```python
from build123d import *

# Parameters (mm, degrees)
SKETCH1_R           = 41
SKETCH1_R_2         = 5
BOSS_EXTRUDE1_DEPTH = 3
SKETCH2_W           = 11
SKETCH2_H           = 12
BOSS_EXTRUDE2_DEPTH = 25
SKETCH3_W           = 7
SKETCH3_H           = 8
CUT_EXTRUDE1_DEPTH  = 65.389440128
SKETCH4_W           = 3
SKETCH4_H           = 3
CUT_EXTRUDE2_DEPTH  = 69.023892861
BOSS_EXTRUDE3_START = -7
BOSS_EXTRUDE3_DEPTH = 7
SKETCH6_R           = 10
SKETCH6_R_2         = 8
BOSS_EXTRUDE4_DEPTH = 5.5


with BuildPart() as part:
    # Sketch1 → Boss-Extrude1 (new body)
    with BuildSketch(Plane.XY):
        Circle(SKETCH1_R)
        Circle(SKETCH1_R_2, mode=Mode.SUBTRACT)
    extrude(amount=BOSS_EXTRUDE1_DEPTH)

    # Sketch2 → Boss-Extrude2 (add)
    with BuildSketch(Plane.XY.offset(3)):
        with Locations((0, 30)):
            Rectangle(SKETCH2_W, SKETCH2_H)
        with Locations((0, 15.301408404)):
            Rectangle(SKETCH2_W, SKETCH2_H)
    extrude(amount=BOSS_EXTRUDE2_DEPTH)

    # Sketch3 → Cut-Extrude1 (cut, through all)
    with BuildSketch(Plane.XY.offset(28)):
        with Locations((0, 30)):
            Rectangle(SKETCH3_W, SKETCH3_H)
        with Locations((0, 15.301408404)):
            Rectangle(SKETCH3_W, SKETCH3_H)
    extrude(amount=-CUT_EXTRUDE1_DEPTH, mode=Mode.SUBTRACT)

    # Sketch4 → Cut-Extrude2 (cut, through all)
    with BuildSketch(Plane(origin=(5.5, 0, 0), x_dir=(0, 0, -1), z_dir=(1, 0, 0))):
        with Locations((-22.5, 15.301408404)):
            Rectangle(SKETCH4_W, SKETCH4_H)
        with Locations((-22.5, 30)):
            Rectangle(SKETCH4_W, SKETCH4_H)
    extrude(amount=-CUT_EXTRUDE2_DEPTH, mode=Mode.SUBTRACT)

    # Sketch5 → Boss-Extrude3 (add)
    with BuildSketch(Plane.XY.offset(3).offset(BOSS_EXTRUDE3_START)):
        with BuildLine():
            Line((16.484910619, 42.944660385), (14.693085931, 38.276797486))
            ThreePointArc((14.693085931, 38.276797486), (20.5, 35.507041555), (25.802136033, 31.86298442))
            Line((25.802136033, 31.86298442), (28.948711541, 35.748681567))
            ThreePointArc((28.948711541, 35.748681567), (22.999978988, 39.837132179), (16.484910619, 42.944660385))
        make_face()
        with BuildLine():
            Line((45.43362216, 7.195978818), (40.495221964, 6.413813067))
            ThreePointArc((40.495221964, 6.413813067), (41, 0), (40.495221964, -6.413813067))
            Line((40.495221964, -6.413813067), (45.43362216, -7.195978818))
            ThreePointArc((45.43362216, -7.195978818), (45.999957975, 0), (45.43362216, 7.195978818))
        make_face()
        with BuildLine():
            Line((28.948711541, -35.748681567), (25.802136033, -31.86298442))
            ThreePointArc((25.802136033, -31.86298442), (20.5, -35.507041555), (14.693085931, -38.276797486))
            Line((14.693085931, -38.276797486), (16.484910619, -42.944660385))
            ThreePointArc((16.484910619, -42.944660385), (22.999978988, -39.837132179), (28.948711541, -35.748681567))
        make_face()
        with BuildLine():
            Line((-16.484910619, -42.944660385), (-14.693085931, -38.276797486))
            ThreePointArc((-14.693085931, -38.276797486), (-20.5, -35.507041555), (-25.802136033, -31.86298442))
            Line((-25.802136033, -31.86298442), (-28.948711541, -35.748681567))
            ThreePointArc((-28.948711541, -35.748681567), (-22.999978988, -39.837132179), (-16.484910619, -42.944660385))
        make_face()
        with BuildLine():
            Line((-45.43362216, -7.195978818), (-40.495221964, -6.413813067))
            ThreePointArc((-40.495221964, -6.413813067), (-41, 0), (-40.495221964, 6.413813067))
            Line((-40.495221964, 6.413813067), (-45.43362216, 7.195978818))
            ThreePointArc((-45.43362216, 7.195978818), (-45.999957975, 0), (-45.43362216, -7.195978818))
        make_face()
        with BuildLine():
            Line((-28.948711541, 35.748681567), (-25.802136033, 31.86298442))
            ThreePointArc((-25.802136033, 31.86298442), (-20.5, 35.507041555), (-14.693085931, 38.276797486))
            Line((-14.693085931, 38.276797486), (-16.484910619, 42.944660385))
            ThreePointArc((-16.484910619, 42.944660385), (-22.999978988, 39.837132179), (-28.948711541, 35.748681567))
        make_face()
    extrude(amount=BOSS_EXTRUDE3_DEPTH)

    # Sketch6 → Boss-Extrude4 (add)
    with BuildSketch(Plane.XY.offset(3)):
        Circle(SKETCH6_R)
        Circle(SKETCH6_R_2, mode=Mode.SUBTRACT)
    extrude(amount=BOSS_EXTRUDE4_DEPTH)


solid = part.part
```
Could you check a few things on this model? Use its own coordinates, in mm. A direction names the side the tool comes from. Coordinates: 2 decimals unless noted, no trailing zeros. Loops run counter-clockwise (first coordinate to the right, second up) from the corner with the lowest first, then second, coordinate; pieces in that order, holes last. Notation, with made-up numbers: M 78,57.25 L 87,57.25 A30 ccw 87,87.25 Z; hole C 76,87 d6. An arc over 180 degrees is marked long. Put each result on its own line as item: value. Start each with the question number.
(1) Suppose I cut it at D-D on x = 0. Count the separate pieces of the cut face and the enclosed holes in it, then the cut area to 3 significant figures.
(2) Will these pins go through, and if not, where does the flat tip stop? P1, Ø1.6, axis at x = -4.5, y = 14.5, coming from the -Z side; P2, Ø1.5, axis at x = -6, z = 18.5, coming from the +Y side; P3, Ø3.5, axis at x = 1.5, z = 16.5, coming from the -Y side.
(3) I need wall thicknesses on line 1 (Y direction, x = 0, z = 0.65); line 2 (Y direction, x = 0, z = 5); line 3 (X direction, y = 32.5, z = 14). Which ranges of each line are inside material? Lowest first, please. Write a range as from..to.
(4) Thinking about a two-plate mould opening in Z: for faces 1 (the face through (-4, 30, 28)), 2 (the face through (5, 15, 24)), 3 (the face through (0, 19.301, 14)), which applies, pulls with the +Z half, pulls with the -Z half, needs draft (parallel to the pull), parting line crosses it, or undercut?
(5) Suppose I cut it at B-B on z = 6. Please give me the cut outline in (x, y), then the cut area to 3 significant figures.
(6) Suppose I cut it at C-C on y = 0. Please give me the cut outline in (x, z).
(7) For faces 4 (the face through (27.397, -33.833, -0.549)), 5 (the face through (0, 24, 15)), 6 (the face through (0, 26, 14)), 7 (the face through (-0.8, -8.2, 8.5)), which set-ups out of +Z, -Z, +X, -X, +Y, -Y let a thin tool reach every point of the face, with its end or its side?
(8) Suppose I cut it at A-A on z = 14. Please give me the cut outline in (x, y).
Solutions:
1. separate pieces: 4
1. enclosed holes: 0
1. area: 386 mm2
2. P1: stops at z = 0
2. P2: stops at y = 36
2. P3: stops at y = 9.3
3. line 1: y = -41..-5, 5..11.3, 19.3..26, 34..41
3. line 2: y = -10..-8, 8..11.3, 19.3..21.3, 24..26, 34..36
3. line 3: x = -5.5..-3.5, 3.5..5.5
4. face 1: pulls with the +Z half
4. face 2: undercut
4. face 3: needs draft
5. outline: M -5.5,9.3 L -3.67,9.3 A10 ccw long 3.67,9.3 L 5.5,9.3 L 5.5,21.3 L -5.5,21.3 Z; M -5.5,24 L 5.5,24 L 5.5,36 L -5.5,36 Z; hole C 0,0 d16; hole M -3.5,11.3 L 3.5,11.3 L 3.5,19.3 L -3.5,19.3 Z; hole M -3.5,26 L 3.5,26 L 3.5,34 L -3.5,34 Z
5. area: 262 mm2
6. outline: M -46,-4 L -41,-4 L -41,0 L -5,0 L -5,3 L -8,3 L -8,8.5 L -10,8.5 L -10,3 L -46,3 Z; M 5,0 L 41,0 L 41,-4 L 46,-4 L 46,3 L 10,3 L 10,8.5 L 8,8.5 L 8,3 L 5,3 Z
7. face 4: +Z, -Z, +X
7. face 5: +Z, +X, -X
7. face 6: +Z, -Z
7. face 7: +Z, +X, -X, -Y
8. outline: M -5.5,9.3 L 5.5,9.3 L 5.5,21.3 L -5.5,21.3 Z; M -5.5,24 L 5.5,24 L 5.5,36 L -5.5,36 Z; hole M -3.5,11.3 L 3.5,11.3 L 3.5,19.3 L -3.5,19.3 Z; hole M -3.5,26 L 3.5,26 L 3.5,34 L -3.5,34 Z
